```python
from build123d import *

# Parameters (mm, degrees)
RECTANGLE134_W                               = 40
RECTANGLE134_H                               = 3
EXTRUDE175_DEPTH                             = 3
RECTANGLE135_W                               = 40
RECTANGLE135_H                               = 3
EXTRUDE176_DEPTH                             = 3
RECTANGLE133_W                               = 40
RECTANGLE133_H                               = 3
EXTRUDE174_DEPTH                             = 3
RECTANGLE128_AS_DRAWN_W                      = 25
RECTANGLE128_AS_DRAWN_H                      = 3
EXTRUDE161_DEPTH                             = 3
EXTRUDE161_ONTO_RECTANGLE128_ROLL_ANGLE      = -90
EXTRUDE161_ONTO_RECTANGLE128_PLACEMENT_ANGLE = 180
RECTANGLE129_AS_DRAWN_W                      = 25
RECTANGLE129_AS_DRAWN_H                      = 3
EXTRUDE159_DEPTH                             = 3
EXTRUDE159_ONTO_RECTANGLE129_ROLL_ANGLE      = -90
EXTRUDE159_ONTO_RECTANGLE129_PLACEMENT_ANGLE = 180
RECTANGLE127_AS_DRAWN_W                      = 25
RECTANGLE127_AS_DRAWN_H                      = 3
EXTRUDE151_DEPTH                             = 3
EXTRUDE151_ONTO_RECTANGLE127_ROLL_ANGLE      = -90
EXTRUDE151_ONTO_RECTANGLE127_PLACEMENT_ANGLE = 180
EXTRUDE154_DEPTH                             = 3
EXTRUDE154_ONTO_RECTANGLE129_ROLL_ANGLE      = -90
EXTRUDE154_ONTO_RECTANGLE129_PLACEMENT_ANGLE = 180
BOX036_W                                     = 283
BOX036_H                                     = 155
BOX036_DEPTH                                 = 3


with BuildPart() as extrude175:
    # Rectangle134 → Extrude175 (new body)
    with BuildSketch(Plane(origin=(114, 38, -112), x_dir=(0, 1, 0), z_dir=(1, 0, 0))):
        with Locations((20, -1.5)):
            Rectangle(RECTANGLE134_W, RECTANGLE134_H)
    extrude(amount=EXTRUDE175_DEPTH)


with BuildPart() as extrude176:
    # Rectangle135 → Extrude176 (new body)
    with BuildSketch(Plane(origin=(114, -19.5, -112), x_dir=(0, 1, 0), z_dir=(1, 0, 0))):
        with Locations((20, -1.5)):
            Rectangle(RECTANGLE135_W, RECTANGLE135_H)
    extrude(amount=EXTRUDE176_DEPTH)


with BuildPart() as extrude174:
    # Rectangle133 → Extrude174 (new body)
    with BuildSketch(Plane(origin=(114, -77, -112), x_dir=(0, 1, 0), z_dir=(1, 0, 0))):
        with Locations((20, -1.5)):
            Rectangle(RECTANGLE133_W, RECTANGLE133_H)
    extrude(amount=EXTRUDE174_DEPTH)


with BuildPart() as fusion064047:
    # Fusion064047 base: copy of Extrude174
    add(extrude174.part)

    # Fusion064047: union Extrude175, Extrude176
    add(extrude175.part)
    add(extrude176.part)


with BuildPart() as fusion064047_1:
    # Fusion064047 placement: moved
    add(fusion064047.part.moved(Location((-283, 0, 0))))


with BuildPart() as fusion064041:
    # Fusion064041 base: copy of Extrude174
    add(extrude174.part)

    # Fusion064041: union Extrude175, Extrude176
    add(extrude175.part)
    add(extrude176.part)


with BuildPart() as fusion064041_1:
    # Fusion064041 placement: moved
    add(fusion064041.part.moved(Location((-3, 0, 0))))


with BuildPart() as extrude161:
    # Rectangle128 as drawn → Extrude161 (new)
    with BuildSketch(Plane.XY):
        with Locations((12.5, 1.5)):
            Rectangle(RECTANGLE128_AS_DRAWN_W, RECTANGLE128_AS_DRAWN_H)
    extrude(amount=-EXTRUDE161_DEPTH)


with BuildPart() as extrude161_1:
    # Extrude161 onto Rectangle128 roll: moved
    add(extrude161.part.rotate(Axis((0, 0, 0), (1, 0, 0)), EXTRUDE161_ONTO_RECTANGLE128_ROLL_ANGLE))


with BuildPart() as extrude161_2:
    # Extrude161 onto Rectangle128 placement: moved
    add(extrude161_1.part.moved(Location((89, -77, -70))).rotate(Axis((89, -77, -70), (0, 0, 1)), EXTRUDE161_ONTO_RECTANGLE128_PLACEMENT_ANGLE))


with BuildPart() as extrude161_3:
    # Extrude161 placement: moved
    add(extrude161_2.part.moved(Location((-208, 0, -42))))


with BuildPart() as extrude159:
    # Rectangle129 as drawn → Extrude159 (new)
    with BuildSketch(Plane.XY):
        with Locations((12.5, 1.5)):
            Rectangle(RECTANGLE129_AS_DRAWN_W, RECTANGLE129_AS_DRAWN_H)
    extrude(amount=-EXTRUDE159_DEPTH)


with BuildPart() as extrude159_1:
    # Extrude159 onto Rectangle129 roll: moved
    add(extrude159.part.rotate(Axis((0, 0, 0), (1, 0, 0)), EXTRUDE159_ONTO_RECTANGLE129_ROLL_ANGLE))


with BuildPart() as extrude159_2:
    # Extrude159 onto Rectangle129 placement: moved
    add(extrude159_1.part.moved(Location((64, -77, -70))).rotate(Axis((64, -77, -70), (0, 0, 1)), EXTRUDE159_ONTO_RECTANGLE129_PLACEMENT_ANGLE))


with BuildPart() as extrude159_3:
    # Extrude159 placement: moved
    add(extrude159_2.part.moved(Location((-133, 0, -42))))


with BuildPart() as fusion064034:
    # Fusion064034 base: copy of Extrude159
    add(extrude159_3.part)

    # Fusion064034: union Extrude161
    add(extrude161_3.part)


with BuildPart() as fusion064034_1:
    # Fusion064034 placement: moved
    add(fusion064034.part.moved(Location((0, 152, 0))))


with BuildPart() as extrude151:
    # Rectangle127 as drawn → Extrude151 (new)
    with BuildSketch(Plane.XY):
        with Locations((12.5, 1.5)):
            Rectangle(RECTANGLE127_AS_DRAWN_W, RECTANGLE127_AS_DRAWN_H)
    extrude(amount=-EXTRUDE151_DEPTH)


with BuildPart() as extrude151_1:
    # Extrude151 onto Rectangle127 roll: moved
    add(extrude151.part.rotate(Axis((0, 0, 0), (1, 0, 0)), EXTRUDE151_ONTO_RECTANGLE127_ROLL_ANGLE))


with BuildPart() as extrude151_2:
    # Extrude151 onto Rectangle127 placement: moved
    add(extrude151_1.part.moved(Location((114, -77, -70))).rotate(Axis((114, -77, -70), (0, 0, 1)), EXTRUDE151_ONTO_RECTANGLE127_PLACEMENT_ANGLE))


with BuildPart() as extrude151_3:
    # Extrude151 placement: moved
    add(extrude151_2.part.moved(Location((0, 0, -42))))


with BuildPart() as extrude154:
    # Rectangle129 as drawn → Extrude154 (new)
    with BuildSketch(Plane.XY):
        with Locations((12.5, 1.5)):
            Rectangle(RECTANGLE129_AS_DRAWN_W, RECTANGLE129_AS_DRAWN_H)
    extrude(amount=-EXTRUDE154_DEPTH)


with BuildPart() as extrude154_1:
    # Extrude154 onto Rectangle129 roll: moved
    add(extrude154.part.rotate(Axis((0, 0, 0), (1, 0, 0)), EXTRUDE154_ONTO_RECTANGLE129_ROLL_ANGLE))


with BuildPart() as extrude154_2:
    # Extrude154 onto Rectangle129 placement: moved
    add(extrude154_1.part.moved(Location((64, -77, -70))).rotate(Axis((64, -77, -70), (0, 0, 1)), EXTRUDE154_ONTO_RECTANGLE129_PLACEMENT_ANGLE))


with BuildPart() as extrude154_3:
    # Extrude154 placement: moved
    add(extrude154_2.part.moved(Location((0, 0, -42))))


with BuildPart() as fusion064040:
    # Fusion064033 base: copy of Extrude154
    add(extrude154_3.part)

    # Fusion064033: union Extrude151
    add(extrude151_3.part)


with BuildPart() as fusion064040_1:
    # Fusion064033 placement: moved
    add(fusion064040.part.moved(Location((0, 152, 0))))

    # Fusion064040: union Fusion064034
    add(fusion064034_1.part)


with BuildPart() as fusion064032:
    # Fusion064032 base: copy of Extrude159
    add(extrude159_3.part)

    # Fusion064032: union Extrude161
    add(extrude161_3.part)


with BuildPart() as fusion064029:
    # Fusion064029 base: copy of Extrude154
    add(extrude154_3.part)

    # Fusion064029: union Extrude151
    add(extrude151_3.part)


with BuildPart() as base_lower003:
    # Box036 → Box036 (new body)
    with BuildSketch(Plane(origin=(-169, -77, -115), x_dir=(1, 0, 0), z_dir=(0, 0, 1))):
        with Locations((141.5, 77.5)):
            Rectangle(BOX036_W, BOX036_H)
    extrude(amount=BOX036_DEPTH)

    # Cut035018: cut Fusion064029
    add(fusion064029.part, mode=Mode.SUBTRACT)

    # Cut035022: cut Fusion064032
    add(fusion064032.part, mode=Mode.SUBTRACT)

    # Cut035027: cut Fusion064040
    add(fusion064040_1.part, mode=Mode.SUBTRACT)

    # Cut035029: cut Fusion064041
    add(fusion064041_1.part, mode=Mode.SUBTRACT)

    # Cut035033: cut Fusion064047
    add(fusion064047_1.part, mode=Mode.SUBTRACT)


with BuildPart() as base_lower003_1:
    # Cut035033 placement: moved
    add(base_lower003.part.moved(Location((0, 0, -4))))


solid = base_lower003_1.part
```
Part model, mm, in its own coordinate system. Coordinates: 2 decimals unless noted, no trailing zeros. Order: outer loops, then holes, each group sorted by start corner. A loop starts at its lowest first (then second) coordinate and runs counter-clockwise, first axis right, second up. Notation, with made-up numbers: (86.25, 58.25) - (105.25, 58.25) arc R21 ccw to (105.25, 78.25) - close; hole circle Ø6 at (64, 57). An arc over 180 degrees is marked (long way). Return JSON: item names as keys, results as strings. Group by question number.
Item 1: Cut at A-A (x = -75.5). List the corners of the cut face in (y, z), plus the area to 3 significant figures.
Item 2: Cut at B-B (y = 15). List the corners of the cut face in (x, z).
Item 3: Pin check, flat tips, straight feed: pin 1 (1.5 mm diameter, centred on y = 76.5, z = -117, fed in from +X); pin 2 (0.9 mm diameter, centred on x = 113, z = -117, fed in from +Y); pin 3 (1.5 mm diameter, centred on y = -53, z = -117.5, fed in from +X). Stop position of each tip, or through.
Item 4: Drill centre lines: probe 1 along Y at (x, z) = (42.5, -116.7); probe 2 along X at (y, z) = (-2, -116.3). Where is each one in solid material? Low to high. Write a range as from..to.
Check values:
{
 "1": {"outline": "(-74, -119) - (75, -119) - (75, -116) - (-74, -116) - close", "area": "447 mm2"},
 "2": {"outline": "(-166, -119) - (111, -119) - (111, -116) - (-166, -116) - close"},
 "3": {"pin 1": "stops at x = 89", "pin 2": "stops at y = 38", "pin 3": "stops at x = 111"},
 "4": {"probe 1": "y = -74..75", "probe 2": "x = -166..111"}
}
